Autodesk Inventor part; units mm, degrees
ref_plane "Start plane" through (0, 0, 0) normal (0, 0, 1) x (1, 0, 0)
ref_plane "End plane" through (0, 0, 1555) normal (0, 0, 1) x (1, 0, 0)
ref_plane "Work Plane4" through (55, 0, 1555) normal (-0.7071, 0, 0.7071) x (0.7071, 0, 0.7071)
ref_plane "Start plane" through (0, 0, 0) normal (0, 0, 1) x (1, 0, 0)
ref_plane "End plane" through (0, 0, 1555) normal (0, 0, 1) x (1, 0, 0)
sketch "Sketch2" plane through (0, 0, 0) normal (0, 0, 1) x (1, 0, 0)
  line L0 (-55, 100.8) -> (-14.95, 100.8)
  line L1 (-55, 110) -> (-55, 100.8)
  line L2 (55, 110) -> (-55, 110)
  line L3 (55, 100.8) -> (55, 110)
  line L4 (14.95, 100.8) -> (55, 100.8)
  line L5 (2.95, -88.8) -> (2.95, 88.8)
  line L6 (55, -100.8) -> (14.95, -100.8)
  line L7 (55, -110) -> (55, -100.8)
  line L8 (-55, -100.8) -> (-55, -110)
  line L9 (-14.95, -100.8) -> (-55, -100.8)
  line L10 (-2.95, 88.8) -> (-2.95, -88.8)
  line L11 (0, -154) -> (0, 154) construction
  line L12 (-2.95, -100.8) -> (2.95, -100.8) construction
  arc A0 (-14.95, -100.8) -> (-2.95, -88.8) centre (-14.95, -88.8) ccw
  arc A1 (-2.95, 88.8) -> (-14.95, 100.8) centre (-14.95, 88.8) ccw
  arc A2 (14.95, 100.8) -> (2.95, 88.8) centre (14.95, 88.8) ccw
  arc A3 (2.95, -88.8) -> (14.95, -100.8) centre (14.95, -88.8) ccw
  line L13 (-77, 0) -> (77, 0) construction
  line L14 (-55, -110) -> (55, -110)
  point P0 (-2.95, 100.8)
  point P1 (2.95, 100.8)
  point P2 (0, 0)
  point P3 (0, -100.8)
  point P4 (0, 0)
  dimension "d1" = 220
  dimension "d3" = 9.2
  dimension "d5" = 5.9
  dimension "d7" = 110
  dimension "d13" = 12
  dimension "d14" = 110
  dimension "d15" = 55
extrude "Body" add sketch "Sketch2" along normal up to surface (1555 mm away) from surface at 0
sketch "Sketch3" plane through (0, 0, 0) normal (0, 0, 1) x (1, 0, 0)
  line L0 (0, 0) -> (10, 0)
ref_plane "Work Plane3" through (0, 0, 0) normal (0, -1, 0) x (1, 0, 0)
ref_plane "Work Plane4" through (55, 0, 1555) normal (-0.7071, 0, 0.7071) x (0.7071, 0, 0.7071)
split "Split1" plane through (55, 0, 1555) removes the side toward (-0.7071, 0, 0.7071)
sketch "Sketch4" plane through (0, 0, 0) normal (0, -1, 0) x (1, 0, 0)
  line L0 (-2, 0) -> (12, 0)
  line L1 (-2, 1555) -> (12, 1555)
  dimension "d19" = 1555
equation "\"d1\" = ParH"
equation "\"d3\" = t2"
equation "\"d7\" = b"
equation "\"d13\" = R1"
equation "\"d14\" = 0.5 * d1"
equation "\"d15\" = 0.5 * d7"
equation "\"d8\" = G_L"
equation "\"b\" = 110"
equation "\"ParH\" = 220"
equation "\"R1\" = 12"
equation "\"G_L\" = d19"
equation "\"t1\" = 5.9"
equation "\"t2\" = 9.2"
equation "\"G_OFFSET_START\" = 0"
equation "\"G_OFFSET_END\" = 55"
equation "\"d17\" = G_OFFSET_END + B_L"
properties part number "DIN 1025 - IPE 220-1555" material "Steel, Mild"
Read the model definition and answer for the solid it produces. Units are mm, in the model's axes. A direction names the side the tool comes from. Coordinates: 2 decimals unless noted, no trailing zeros. Write each loop counter-clockwise with the first axis right and the second up, starting at its lowest first coordinate (ties: lowest second). Pieces come first, ordered by that corner, then holes. Notation, with made-up numbers: (51.5, 23) - (97.5, 23) arc R18 cw to (97.5, 42) - close; hole circle Ø8 at (-6, 39). An arc over 180 degrees is marked (long way). Answer as a JSON object with one key per item and string values. Group by question number.
1. A cutting plane is placed at A-A (x = 33). Determine the outline of the cut face in (y, z).
2. Each of these flat-tipped pins is pushed along its axis until it touches: P1, Ø3, axis at y = -45, z = 1131, coming from the +X side; P2, Ø8, axis at y = 47.5, z = 1019.5, coming from the -X side. Where does it stop, or does it pass through?
3. Which of the six approach directions +Z, -Z, +X, -X, +Y, -Y give full straight-line access (tool end or side, diameter ignored) to faces 4 (the flat face through (2.95, -1, 741)), 5 (the flat face through (0, -1, 1500)), 6 (the flat face through (-35, -100.8, 732))?
4. The mould has two halves that part along Y. Classify faces 1 (the flat face through (-35, 100.8, 732)), 2 (the flat face through (-1, -110, 767)), 3 (the flat face through (0, 1, 0)): +Y half, -Y half, draft (parallel to the pull), parting line (faces both ways), or undercut.
5. A cutting plane is placed at C-C (y = 34). Determine the outline of the cut face in (x, z).
6. Consider L1, parallel to Y at x = -17.5, z = 62; L2, parallel to X at y = 57.5, z = 1238; L3, parallel to Y at x = -10, z = 728. Determine where each line is inside the solid, lowest interval first. Write a range as [from, to].
7. A cutting plane is placed at B-B (z = 624). Determine the outline of the cut face in (x, y), plus the area to 3 significant figures.
Worked out:
{
 "1": {"outline": "(-110, 0) - (-100.8, 0) - (-100.8, 1533) - (-110, 1533) - close; (100.8, 0) - (110, 0) - (110, 1533) - (100.8, 1533) - close"},
 "2": {"P1": "stops at x = 2.95", "P2": "stops at x = -2.95"},
 "3": {"face 4": "+Z, -Z, +X", "face 5": "+Z, -X, +Y, -Y", "face 6": "+Z, -Z, -X"},
 "4": {"face 1": "undercut", "face 2": "-Y half", "face 3": "draft"},
 "5": {"outline": "(-2.95, 0) - (2.95, 0) - (2.95, 1502.95) - (-2.95, 1497.05) - close"},
 "6": {"L1": "y = [-110, -100.8], [100.8, 110]", "L2": "x = [-2.95, 2.95]", "L3": "y = [-110, -99.73], [99.73, 110]"},
 "7": {"outline": "(-55, -110) - (55, -110) - (55, -100.8) - (14.95, -100.8) arc R12 cw to (2.95, -88.8) - (2.95, 88.8) arc R12 cw to (14.95, 100.8) - (55, 100.8) - (55, 110) - (-55, 110) - (-55, 100.8) - (-14.95, 100.8) arc R12 cw to (-2.95, 88.8) - (-2.95, -88.8) arc R12 cw to (-14.95, -100.8) - (-55, -100.8) - close", "area": "3,340 mm²"}
}
